Model file for the job. Use its own axes, mm. Face numbers are marked on the shaded views. A direction names the side the tool comes from. Give positions to 0.01 mm unless a question says otherwise; leave off trailing zeros. Loops run counter-clockwise (first coordinate to the right, second up) from the corner with the lowest first, then second, coordinate; pieces in that order, holes last. Notation, with made-up numbers: (-16, -19.75) - (30, -19.75) arc R24 cw to (30, 11.25) - close; hole circle Ø5 at (45.5, 20). An arc over 180 degrees is marked (long way). Answer as CSV lines item,"result". Start each with the question number.
Item 1: Tool access for the marked faces 1, 2 and 3: list every direction of +Z, -Z, +X, -X, +Y, -Y with a clear straight run to the whole face (end or side of a thin tool).
Item 2: Saw through at C-C on x = 283.5. Give the cut face in (y, z).
Item 3: Saw through at A-A on y = 0. Give the cut face in (x, z), plus the area to 3 significant figures.
Item 4: Pin check, flat tips, straight feed: pin 1 (5 mm diameter, centred on x = 398.5, y = 59, fed in from -Z); pin 2 (3 mm diameter, centred on x = 391, z = 1, fed in from +Y); pin 3 (10.5 mm diameter, centred on x = 62.5, y = 49, fed in from +Z). Stop position of each tip, or through.
Item 5: Drill centre lines: L1, parallel to Z at x = 384.5, y = 2.5; L2, parallel to X at y = -39, z = 49.5; L3, parallel to Z at x = 210, y = 2.5. Where is each one in solid material? Low to high. Write a range as from..to.
Item 6: Saw through at B-B on z = 0. Give the cut face in (x, y), plus the area to 3 significant figures.
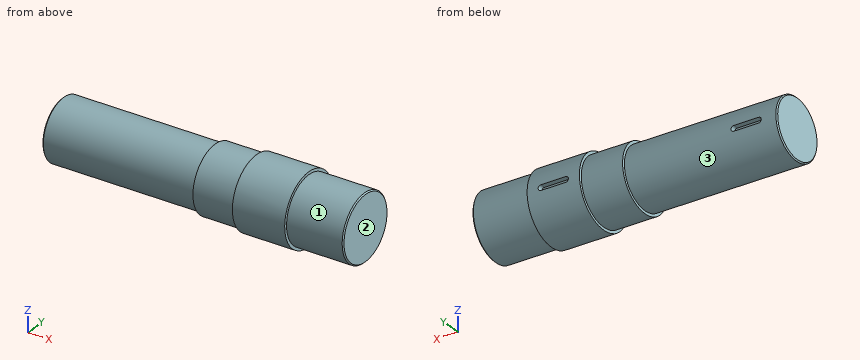
from build123d import *

# Parameters (mm, degrees)
CHAFL_N1_SIZE         = 2
CHAFL_N2_SIZE         = 2
CORTAR_EXTRUIR1_DEPTH = 10
CORTAR_EXTRUIR2_DEPTH = 10


with BuildPart() as part:
    # Croquis1 → Revolución2 (revolve)
    with BuildSketch(Plane(origin=(0, 0, 0), x_dir=(1, 0, 0), z_dir=(0, 1, 0)), mode=Mode.PRIVATE) as revoluci_n2_sk:
        Polygon((0, 0), (550, 0), (550, 60), (447, 60), (447, 65), (352, 65), (352, 60), (277, 60), (277, 55), (0, 55), align=None)
    revolve(revoluci_n2_sk.sketch.rotate(Axis((0, 0, 0), (1, 0, 0)), 180), axis=Axis((0, 0, 0), (1, 0, 0)))

    # Chaflán1
    chafl_n1_edges = [part.edges().sort_by_distance(p)[0] for p in [
        (0, 0, -55),
    ]]
    chamfer(chafl_n1_edges, length=CHAFL_N1_SIZE)

    # Chaflán2
    chafl_n2_edges = [part.edges().sort_by_distance(p)[0] for p in [
        (550, 0, -60),
    ]]
    chamfer(chafl_n2_edges, length=CHAFL_N2_SIZE)

    # Croquis2 → Cortar-Extruir1 (cut)
    with BuildSketch(Plane(origin=(0, 65, 0), x_dir=(1, 0, 0), z_dir=(0, 1, 0))):
        with BuildLine():
            Line((377, -5), (422, -5))
            ThreePointArc((422, -5), (427, 0), (422, 5))
            Line((422, 5), (377, 5))
            ThreePointArc((377, 5), (372, 0), (377, -5))
        make_face()
    extrude(amount=-CORTAR_EXTRUIR1_DEPTH, mode=Mode.SUBTRACT)

    # Croquis3 → Cortar-Extruir2 (cut)
    with BuildSketch(Plane(origin=(0, 55, 0), x_dir=(1, 0, 0), z_dir=(0, 1, 0))):
        with BuildLine():
            Line((33.490249976, -5), (78.490249976, -5))
            ThreePointArc((78.490249976, -5), (83.490249976, 0), (78.490249976, 5))
            Line((78.490249976, 5), (33.490249976, 5))
            ThreePointArc((33.490249976, 5), (28.490249976, 0), (33.490249976, -5))
        make_face()
    extrude(amount=-CORTAR_EXTRUIR2_DEPTH, mode=Mode.SUBTRACT)


solid = part.part
Responses:
1,face 1,"+X"
1,face 2,"+Z, -Z, +X, +Y, -Y"
1,face 3,"-X"
2,outline,"circle Ø120 at (0, 0)"
3,outline,"(0, -53) - (2, -55) - (277, -55) - (277, -60) - (352, -60) - (352, -65) - (447, -65) - (447, -60) - (548, -60) - (550, -58) - (550, 58) - (548, 60) - (447, 60) - (447, 65) - (352, 65) - (352, 60) - (277, 60) - (277, 55) - (2, 55) - (0, 53) - close"
3,area,"64,200 mm2"
4,pin 1,"z = -32.14"
4,pin 2,"y = 55"
4,pin 3,"z = 33.33"
5,L1,"-64.95..64.95"
5,L2,"352..447"
5,L3,"-54.94..54.94"
6,outline,"(0, -53) - (2, -55) - (277, -55) - (277, -60) - (352, -60) - (352, -65) - (447, -65) - (447, -60) - (548, -60) - (550, -58) - (550, 58) - (548, 60) - (447, 60) - (447, 65) - (427, 65) - (427, 55) - (372, 55) - (372, 65) - (352, 65) - (352, 60) - (277, 60) - (277, 55) - (83.49, 55) - (83.49, 45) - (28.49, 45) - (28.49, 55) - (2, 55) - (0, 53) - close"
6,area,"63,100 mm2"
